from build123d import *

# Parameters (mm, degrees)
BOSS_EXTRUDE3_DEPTH = 3
MOVE_FACE1_BY       = 5.4
SKETCH3_W           = 115
SKETCH3_H           = 46.6
BOSS_EXTRUDE4_DEPTH = 3
FILLET3_R           = 5
FILLET5_R           = 2
SKETCH4_R           = 1.15
CUT_EXTRUDE1_DEPTH  = 134.861204865
SKETCH5_R           = 1.2
CUT_EXTRUDE2_DEPTH  = 154.25224305
SKETCH6_R           = 1.15
CUT_EXTRUDE6_DEPTH  = 134.861205025


with BuildPart() as part:
    # Sketch1 → Boss-Extrude3 (new body)
    with BuildSketch(Plane.XY):
        with BuildLine():
            Line((-49.5, -25.454214411), (49.5, -25.454214411))
            ThreePointArc((49.5, -25.454214411), (55.156854249, -23.111068661), (57.5, -17.454214411))
            Line((57.5, -17.454214411), (57.5, 104.345785589))
            Line((57.5, 104.345785589), (-57.5, 104.345785589))
            Line((-57.5, 104.345785589), (-57.5, -17.454214411))
            ThreePointArc((-57.5, -17.454214411), (-55.156854249, -23.111068661), (-49.5, -25.454214411))
        make_face()
    extrude(amount=BOSS_EXTRUDE3_DEPTH)

    # Move Face1: a face moved outward by 5.4
    extrude(part.faces().sort_by_distance((0, 104.345785589, 1.5))[0], amount=MOVE_FACE1_BY, dir=(0, 1, 0))

    # Sketch3 → Boss-Extrude4 (add)
    with BuildSketch(Plane(origin=(0, 109.745785589, 0), x_dir=(1, 0, 0), z_dir=(0, 1, 0))):
        with Locations((0, 20.3)):
            Rectangle(SKETCH3_W, SKETCH3_H)
    extrude(amount=BOSS_EXTRUDE4_DEPTH)

    # Fillet3
    fillet3_edges = [part.edges().sort_by_distance(p)[0] for p in [
        (0, 109.745785589, 0),
    ]]
    fillet(fillet3_edges, radius=FILLET3_R)

    # Fillet5
    fillet5_edges = [part.edges().sort_by_distance(p)[0] for p in [
        (-57.5, 112.745785589, -20.3),
        (0, 112.745785589, 3),
        (57.5, 112.745785589, -20.3),
    ]]
    fillet(fillet5_edges, radius=FILLET5_R)

    # Sketch4 → Cut-Extrude1 (cut, through all)
    with BuildSketch(Plane(origin=(0, 0, 0), x_dir=(-1, 0, 0), z_dir=(0, 0, -1))):
        with Locations((-53, -20.954214411)):
            Circle(SKETCH4_R)
        with Locations((-55.25, 44.545785589)):
            Circle(SKETCH4_R)
        with Locations((-55.25, 94.545785589)):
            Circle(SKETCH4_R)
        with Locations((0, -23.454214411)):
            Circle(SKETCH4_R)
        with Locations((53, -20.954214411)):
            Circle(SKETCH4_R)
        with Locations((55.25, 44.545785589)):
            Circle(SKETCH4_R)
        with Locations((55.25, 94.545785589)):
            Circle(SKETCH4_R)
    extrude(amount=-CUT_EXTRUDE1_DEPTH, mode=Mode.SUBTRACT)

    # Sketch5 → Cut-Extrude2 (cut, through all)
    with BuildSketch(Plane.XZ.offset(-109.745785589)):
        with Locations(Location((55.25, -8, 0), (0, 0, 270))):
            Circle(SKETCH5_R)
        with Locations(Location((55.25, -41.8, 0), (0, 0, 270))):
            Circle(SKETCH5_R)
        with Locations(Location((0, -41.8, 0), (0, 0, 270))):
            Circle(SKETCH5_R)
        with Locations(Location((-55.25, -8, 0), (0, 0, 270))):
            Circle(SKETCH5_R)
        with Locations(Location((-55.25, -41.8, 0), (0, 0, 270))):
            Circle(SKETCH5_R)
    extrude(amount=-CUT_EXTRUDE2_DEPTH, mode=Mode.SUBTRACT)

    # Sketch6 → Cut-Extrude6 (cut, through all)
    with BuildSketch(Plane(origin=(0, 0, 0), x_dir=(-1, 0, 0), z_dir=(0, 0, -1))):
        with Locations((-16.5, 46)):
            Circle(SKETCH6_R)
        with Locations((16.5, 46)):
            Circle(SKETCH6_R)
        with Locations((16.5, 94.5)):
            Circle(SKETCH6_R)
        with Locations((-16.5, 94.5)):
            Circle(SKETCH6_R)
    extrude(amount=-CUT_EXTRUDE6_DEPTH, mode=Mode.SUBTRACT)


solid = part.part
Can you work these out from the model? Positions are in its coordinate system, mm. A direction names the side the tool comes from. Coordinates: 2 decimals unless noted, no trailing zeros. Loops run counter-clockwise (first coordinate to the right, second up) from the corner with the lowest first, then second, coordinate; pieces in that order, holes last. Notation, with made-up numbers: (-9.75, 64.5) - (34.25, 64.5) arc R15 cw to (34.25, 81.5) - close; hole circle Ø8 at (-25.75, 87). An arc over 180 degrees is marked (long way). Answer as a JSON object with one key per item and string values. Group by question number.
Item 1: If we section it at B-B (z = -18.5): List the corners of the cut face in (x, y) for me, plus the area to 3 significant figures.
Item 2: If I drill on L1, parallel to Z at x = -55.25, y = 110.8; L2, parallel to Y at x = 0, z = 1.25; L3, parallel to Y at x = -16.5, z = 2.45, over which ranges is the centre line in solid material (lowest first)? Write a range as from..to.
Item 3: If we section it at C-C (y = 99): List the corners of the cut face in (x, z) for me.
Item 4: On a 3-axis mill with a long thin cutter (end or side, diameter ignored), from which of +Z, -Z, +X, -X, +Y, -Y can I reach the whole of each face in a straight line? I mean faces 1 (the face through (-1, 109.746, -25)), 2 (the face through (-55.22, -23.05, 1.48)). Say none if no direction works.
Item 5: For pin 1 (3.5 mm diameter, centred on x = 0, y = -23.45, fed in from -Z); pin 2 (3 mm diameter, centred on x = 55.25, z = -8, fed in from +Y); pin 3 (1 mm diameter, centred on x = -18, z = -4, fed in from -Y); pin 4 (3 mm diameter, centred on x = 0, z = -41.8, fed in from -Y), each with a flat end and sliding along its axis, tell me the tip position at first contact or that it passes through.
Item 6: If we section it at A-A (x = 13): List the corners of the cut face in (y, z) for me, plus the area to 3 significant figures.
Returned:
{
 "1": {"outline": "(-57.5, 109.75) - (57.5, 109.75) - (57.5, 110.75) arc R2 ccw to (55.5, 112.75) - (-55.5, 112.75) arc R2 ccw to (-57.5, 110.75) - close", "area": "343 mm²"},
 "2": {"L1": "z = -43.6..-43, -40.6..-9.2, -6.8..3", "L2": "y = -25.45..-24.6, -22.3..112.73", "L3": "y = -25.45..44.85, 47.15..93.35, 95.65..112.12"},
 "3": {"outline": "(-57.5, 0) - (57.5, 0) - (57.5, 3) - (-57.5, 3) - close"},
 "4": {"face 1": "-Z, +X, -X, -Y", "face 2": "+Z, -Z, -X, -Y"},
 "5": {"pin 1": "stops at z = 0", "pin 2": "stops at y = 112.75", "pin 3": "stops at y = 109.52", "pin 4": "stops at y = 109.75"},
 "6": {"outline": "(-25.45, 0) - (104.75, 0) arc R5 cw to (109.75, -5) - (109.75, -43.6) - (112.75, -43.6) - (112.75, 1) arc R2 ccw to (110.75, 3) - (-25.45, 3) - close", "area": "550 mm²"}
}
